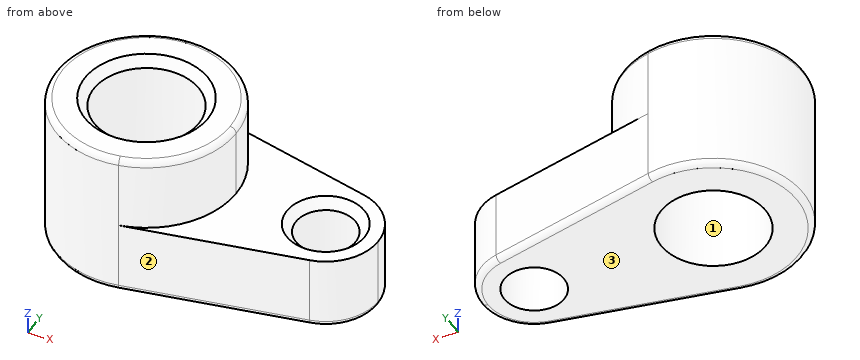
```python
from build123d import *

# Parameters (mm, degrees)
F0_R     = 17.5
F0_R_2   = 10
F1_DEPTH = 25
F2_DEPTH = 50
F3_R     = 2
F4_SIZE  = 3


with BuildPart() as f1:
    # F0 (on Top) → F1 (new body)
    with BuildSketch(Plane.XY):
        with BuildLine():
            ThreePointArc((6.25, -29.341736), (23.318448, -18.874586), (30, 0))
            ThreePointArc((30, 0), (23.318448, 18.874586), (6.25, 29.341736))
            ThreePointArc((6.25, 29.341736), (-30, 0), (6.25, -29.341736))
        make_face()
        Circle(F0_R, mode=Mode.SUBTRACT)
        with BuildLine():
            ThreePointArc((6.25, 29.341736), (23.318448, 18.874586), (30, 0))
            ThreePointArc((30, 0), (23.318448, -18.874586), (6.25, -29.341736))
            Line((6.25, -29.341736), (63.645833, -17.116013))
            ThreePointArc((63.645833, -17.116013), (42.5, 0), (63.645833, 17.116013))
            Line((63.645833, 17.116013), (6.25, 29.341736))
        make_face()
        with BuildLine():
            ThreePointArc((77.5, 0), (73.602428, 11.010175), (63.645833, 17.116013))
            ThreePointArc((63.645833, 17.116013), (42.5, 0), (63.645833, -17.116013))
            ThreePointArc((63.645833, -17.116013), (73.602428, -11.010175), (77.5, 0))
        make_face()
        with Locations((60, 0)):
            Circle(F0_R_2, mode=Mode.SUBTRACT)
    extrude(amount=F1_DEPTH)

    # F0 (on Top) → F2 (join)
    with BuildSketch(Plane.XY):
        with BuildLine():
            ThreePointArc((6.25, -29.341736), (23.318448, -18.874586), (30, 0))
            ThreePointArc((30, 0), (23.318448, 18.874586), (6.25, 29.341736))
            ThreePointArc((6.25, 29.341736), (-30, 0), (6.25, -29.341736))
        make_face()
        Circle(F0_R, mode=Mode.SUBTRACT)
    extrude(amount=F2_DEPTH)

    # F3
    f3_edges = [f1.edges().sort_by_distance(p)[0] for p in [
        (-6.25, 29.341736, 50),
        (34.947917, -23.228875, 0),
        (34.947917, 23.228875, 0),
    ]]
    fillet(f3_edges, radius=F3_R)

    # F4
    f4_edges = [f1.edges().sort_by_distance(p)[0] for p in [
        (-17.5, 0, 50),
        (50, 0, 25),
    ]]
    chamfer(f4_edges, length=F4_SIZE)


solid = f1.part
```
Check sheet for the modelled part. Datum: model origin and axes. Units: mm. Face numbers are marked on the shaded views. Coordinates: 2 decimals unless noted, no trailing zeros. Order: outer loops, then holes, each group sorted by start corner. A loop starts at its lowest first (then second) coordinate and runs counter-clockwise, first axis right, second up. Notation, with made-up numbers: M 54.25,70 L 96.25,70 A8 ccw 96.25,82 Z; hole C 62,-10 d5. An arc over 180 degrees is marked long. Write each question's results on one line, items separated by ' | '. Start each with the question number.
1. Material ranges on probe 1 along Y at (x, z) = (0, 12); probe 2 along Y at (x, z) = (60, 13); probe 3 along X at (y, z) = (19, 34.5), recorded low to high.
2. Mould release check, pull along X, two halves, no side actions. Record for the marked faces 1, 2 and 3: +X half, -X half, draft (parallel to the pull), parting line (faces both ways), or undercut.
3. Go/stop test with flat-tipped pins: P1, Ø10, axis at x = 40.5, z = 23.5, coming from the +Y side; P2, Ø6, axis at y = -2.5, z = 35, coming from the +X side; P3, Ø3, axis at x = 36.5, z = 13.5, coming from the +Y side. Record where each tip stops, or that it passes through.
4. Cross-section at A-A on z = 16. Record the cut outline in (x, y), and give its area (3 significant figures).
5. Cross-section at B-B on z = 37. Record the cut outline in (x, y), and give its area (3 significant figures).
Checks:
1) probe 1: y = -30 to -17.5, 17.5 to 30 | probe 2: y = -17.89 to -10, 10 to 17.89 | probe 3: x = -23.22 to 23.22
2) face 1: undercut | face 2: +X half | face 3: draft
3) P1: stops at y = 23.11 | P2: stops at x = 30 | P3: stops at y = 23.22
4) outline: M 6.25,-29.34 L 63.65,-17.12 A17.5 ccw 63.65,17.12 L 6.25,29.34 A30 ccw long Z; hole C 0,0 d35; hole C 60,0 d20 | area: 3,530 mm²
5) outline: M 6.25,-29.34 A30 ccw 30,0 A30 ccw 6.25,29.34 A30 ccw long Z; hole C 0,0 d35 | area: 1,870 mm²
